Autodesk Inventor part; units mm, degrees
ref_plane "YZ Plane" through (0, 0, 0) normal (1, 0, 0) x (0, 1, 0)
ref_plane "XZ Plane" through (0, 0, 0) normal (0, 1, 0) x (-1, 0, 0)
ref_plane "XY Plane" through (0, 0, 0) normal (0, 0, 1) x (1, 0, 0)
sketch "Sketch1" plane through (0, 0, 0) normal (1, 0, 0) x (0, 1, 0)
  line L0 (0, 0) -> (-44.5, 0)
  line L1 (-44.5, 0) -> (-44.5, -18)
  line L2 (-44.5, -18) -> (-39.5, -18)
  line L3 (-39.5, -18) -> (-39.5, -5)
  line L4 (-39.5, -5) -> (-3, -5)
  line L5 (-3, -5) -> (-3, -27)
  line L6 (-3, -27) -> (0, -27)
  line L7 (0, -27) -> (0, 0)
  dimension "d0" = 3
  dimension "d1" = 44.5
  dimension "d2" = 5
  dimension "d3" = 27
  dimension "d4" = 18
  dimension "d5" = 5
extrude "Extrusion1" add sketch "Sketch1" along normal blind 20
fillet "Fillet1" radius 4 2 edges at (10, -44.5, 0) (10, -44.5, -18)
chamfer "Chamfer1" distance 4 angle 45 1 edges at (10, -3, -5)
sketch "Sketch2" plane through (0, 0, 0) normal (0, 1, 0) x (1, 0, 0)
  circle A0 centre (10, 13) radius 1.6
  circle A1 centre (10, 23) radius 1.6
  line L0 (0, 0) -> (20, 0) construction
  line L1 (10, 0) -> (10, 27) construction
  line L2 (0, 27) -> (20, 27) construction
  dimension "d12" = 3.2
  dimension "d13" = 13
  dimension "d14" = 10
extrude "Extrusion2" cut sketch "Sketch2" against normal up to surface (3 mm away)
properties part number "Front_Skit_Plate"
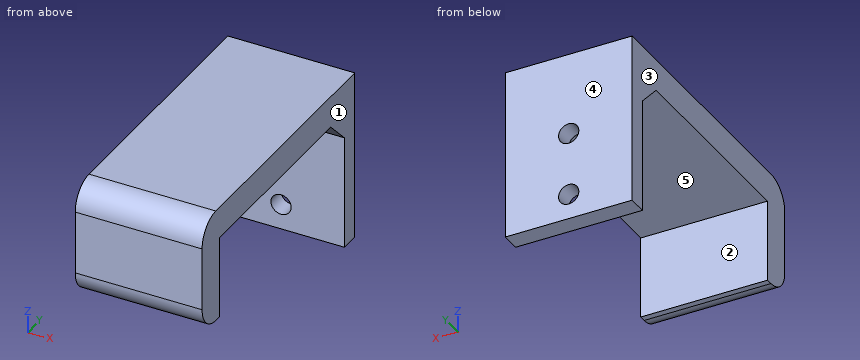
Geometry check sheet. Reference: the model listing, model coordinates, mm. Face numbers are marked on the shaded views. A direction names the side the tool comes from. Coordinates: 2 decimals unless noted, no trailing zeros. Order: outer loops, then holes, each group sorted by start corner. A loop starts at its lowest first (then second) coordinate and runs counter-clockwise, first axis right, second up. Notation, with made-up numbers: (87, -20) - (135, -20) arc R24 ccw to (135, -5) - close; hole circle Ø6 at (35.25, -34). An arc over 180 degrees is marked (long way). Answer as a JSON object with one key per item and string values. Group by question number.
Item 1: Sectioned sample at A-A, the plane z = -6. Record the cut outline in (x, y), and give its area (3 significant figures).
Item 2: Draft check along Y on the marked faces 3, 4 and 5. Enter one of: +Y half, -Y half, draft (parallel to the pull), parting line (faces both ways), or undercut.
Item 3: Scan lines: probe 1 along Z at (x, y) = (10, -1.4); probe 2 along X at (y, z) = (-1.25, -13); probe 3 along Y at (x, z) = (6.5, -24.25). Record each from-to range of solid material in increasing order.
Item 4: Depth check by flat-ended pin: pin 1 Ø10 at (x, y) = (16, -6.5) entering from -Z; pin 2 Ø10 at (x, y) = (13, -25) entering from -Z; pin 3 Ø6 at (y, z) = (-36, -10) entering from -X; pin 4 Ø3 at (x, y) = (7.5, -8) entering from -Z. Enter the tip coordinate at first touch or a pass-through.
Item 5: Tool access check on the marked faces 1 and 2. Record the directions out of +Z, -Z, +X, -X, +Y, -Y that give a thin tool (end or side, any length) a straight path to the whole face; none if there is none.
Item 6: Sectioned sample at C-C, the plane z = -13. Record the cut outline in (x, y), and give its area (3 significant figures).
Item 7: Sectioned sample at B-B, the plane x = 10. Record the cut outline in (y, z).
Item 8: Sectioned sample at D-D, the plane x = 15. Record the cut outline in (y, z), and give its area (3 significant figures).
Resolved:
{
 "1": {"outline": "(0, -44.5) - (20, -44.5) - (20, -39.5) - (0, -39.5) - close; (0, -6) - (20, -6) - (20, 0) - (0, 0) - close", "area": "220 mm^2"},
 "2": {"face 3": "draft", "face 4": "+Y half", "face 5": "undercut"},
 "3": {"probe 1": "-27 to -24.6, -21.4 to -14.6, -11.4 to 0", "probe 2": "0 to 8.4, 11.6 to 20", "probe 3": "-3 to 0"},
 "4": {"pin 1": "z = -27", "pin 2": "z = -5", "pin 3": "through", "pin 4": "z = -5.5"},
 "5": {"face 1": "+Z, -Z, +X, +Y, -Y", "face 2": "-Z, +X, -X"},
 "6": {"outline": "(0, -44.5) - (20, -44.5) - (20, -39.5) - (0, -39.5) - close; (0, -3) - (8.4, -3) - (8.4, 0) - (0, 0) - close; (11.6, -3) - (20, -3) - (20, 0) - (11.6, 0) - close", "area": "150 mm^2"},
 "7": {"outline": "(-44.5, -14) arc R4 ccw to (-40.5, -18) - (-39.5, -18) - (-39.5, -5) - (-7, -5) - (-3, -9) - (-3, -11.4) - (0, -11.4) - (0, 0) - (-40.5, 0) arc R4 ccw to (-44.5, -4) - close; (-3, -27) - (0, -27) - (0, -24.6) - (-3, -24.6) - close; (-3, -21.4) - (0, -21.4) - (0, -14.6) - (-3, -14.6) - close"},
 "8": {"outline": "(-44.5, -14) arc R4 ccw to (-40.5, -18) - (-39.5, -18) - (-39.5, -5) - (-7, -5) - (-3, -9) - (-3, -27) - (0, -27) - (0, 0) - (-40.5, 0) arc R4 ccw to (-44.5, -4) - close", "area": "355 mm^2"}
}
